Geometry: final body of the model. Coordinates: model frame, mm. A direction names the side the tool comes from. Give positions to 0.01 mm unless a question says otherwise; leave off trailing zeros. Loops run counter-clockwise (first coordinate to the right, second up) from the corner with the lowest first, then second, coordinate; pieces in that order, holes last.
1. Section B-B, the plane x = -22.5. Output: boundary loops of the cut face in (y, z).
2. Section D-D, the plane x = 9.5. Output: boundary loops of the cut face in (y, z).
3. Draft query along Z for faces 5 (the face through (0, 0, 39.532)), 6 (the face through (25, 4, 17)), 7 (the face through (28, 0, 16)), 8 (the face through (0, 0, -6.468)). Return one class per face: +Z half, -Z half, draft (parallel to the pull), parting line (faces both ways), or undercut.
4. Section C-C, the plane z = 35. Output: boundary loops of the cut face in (x, y).
5. Access query for faces 1 (the face through (0, 1, 36.532)), 2 (the face through (-25, 4, 16)), 3 (the face through (-0.66, -19.01, 33.73)), 4 (the face through (0, -20, 2)). Directions: +Z, -Z, +X, -X, +Y, -Y. A direction counts if a zero-diameter tool reaches every point of the face in a straight line with its end or side. Return the directions, or none.
6. Material intervals for line 1 along X through (y, z) = (-15, -3); line 2 along Z through (x, y) = (24.5, 5); line 3 along Y through (x, z) = (23.5, 3), sorted ascending.
7. Section A-A, the plane y = -1.5. Output: boundary loops of the cut face in (x, z).
8. First-contact query: P1, Ø24, axis at x = 0, z = 18.74, coming from the -Y side. Flat tip, straight axial feed; report the tip coordinate or a pass-through.
from build123d import *

# Parameters (mm, degrees)
F1_DEPTH = 20
F5_DEPTH = 1
F7_DEPTH = 2


# Not quite as in the source:
# - a feature names something its author has since deleted; it is built from what else it names


with BuildPart() as f1:
    # F0 (on Front) → F1 (new body, symmetric)
    with BuildSketch(Plane.XZ):
        Polygon((-25, -3.4681803342), (-25, 36.5318196658), (25, 36.5318196658), (25, 26.5318196658), (28, 26.5318196658), (28, 39.5318196658), (-28, 39.5318196658), (-28, -6.4681803342), (0, -6.4681803342), (0, -3.4681803342), align=None)
        Polygon((28, 26.5318196658), (25, 26.5318196658), (25, -3.4681803342), (0, -3.4681803342), (0, -6.4681803342), (28, -6.4681803342), align=None)
    extrude(amount=F1_DEPTH, both=True)

    # F4 (on offset) → F5 (join)
    with BuildSketch(Plane.XZ.offset(-20)):
        Polygon((25, -3.5996623058), (25, 36.4003376942), (-25, 36.4003376942), (-25, -3.5996623058), (0, -3.5996623058), align=None)
        with BuildLine():
            ThreePointArc((5, 19.2190613598), (3.5355339059, 15.6835274538), (0, 14.2190613598))
            ThreePointArc((0, 14.2190613598), (-5, 19.2190613598), (0, 24.2190613598))
            ThreePointArc((0, 24.2190613598), (3.5355339059, 22.7545952657), (5, 19.2190613598))
        make_face(mode=Mode.SUBTRACT)
    extrude(amount=F5_DEPTH)

    # F6 (on offset) → F7 (join)
    with BuildSketch(Plane.XZ.offset(20)):
        Polygon((-25, 36.5481637139), (-25, -3.4518362861), (0, -3.4518362861), (25, -3.4518362861), (25, 36.5481637139), align=None)
        with BuildLine():
            ThreePointArc((15, 18.7427662313), (10.6066017178, 8.1361645135), (0, 3.7427662313))
            ThreePointArc((0, 3.7427662313), (-10.6066017178, 29.3493679491), (15, 18.7427662313))
        make_face(mode=Mode.SUBTRACT)
    extrude(amount=-F7_DEPTH)


solid = f1.part
Answers below:
1. outline: (-20, -6.47) - (20, -6.47) - (20, 36.4) - (19, 36.4) - (19, -3.47) - (-20, -3.47) - close; (-20, -3.45) - (-18, -3.45) - (-18, 36.53) - (20, 36.53) - (20, 39.53) - (-20, 39.53) - close
2. outline: (-20, -6.47) - (20, -6.47) - (20, 36.4) - (19, 36.4) - (19, -3.47) - (-20, -3.47) - close; (-20, -3.45) - (-18, -3.45) - (-18, 7.13) - (-20, 7.13) - close; (-20, 30.35) - (-18, 30.35) - (-18, 36.53) - (20, 36.53) - (20, 39.53) - (-20, 39.53) - close
3. face 5: +Z half
3. face 6: undercut
3. face 7: draft
3. face 8: -Z half
4. outline: (-28, -20) - (28, -20) - (28, 20) - (-28, 20) - close; hole (-25, -18) - (25, -18) - (25, 19) - (-25, 19) - close
5. face 1: +Y
5. face 2: none
5. face 3: -Y
5. face 4: +Z, -Z, +X, -X, -Y
6. line 1: x = -28 to -25, 25 to 28
6. line 2: z = -6.47 to -3.47, 36.53 to 39.53
6. line 3: y = -20 to -18, 19 to 20
7. outline: (-28, -6.47) - (28, -6.47) - (28, 39.53) - (-28, 39.53) - close; hole (-25, -3.47) - (25, -3.47) - (25, 36.53) - (-25, 36.53) - close
8. P1: stops at y = 19
